Design review of the part shown in the three views and the two pictorial views. Dimensions are in mm from the part's minimum x, y and z. Give positions to 0.01 mm unless a question says otherwise; leave off trailing zeros. Write each loop counter-clockwise with the first axis right and the second up, starting at its lowest first coordinate (ties: lowest second). Pieces come first, ordered by that corner, then holes. Notation, with made-up numbers: M 42.5,31 L 85.5,31 A22 cw 85.5,44 Z; hole C -13,-19.5 d8. An arc over 180 degrees is marked long. Write item = value, one per line.
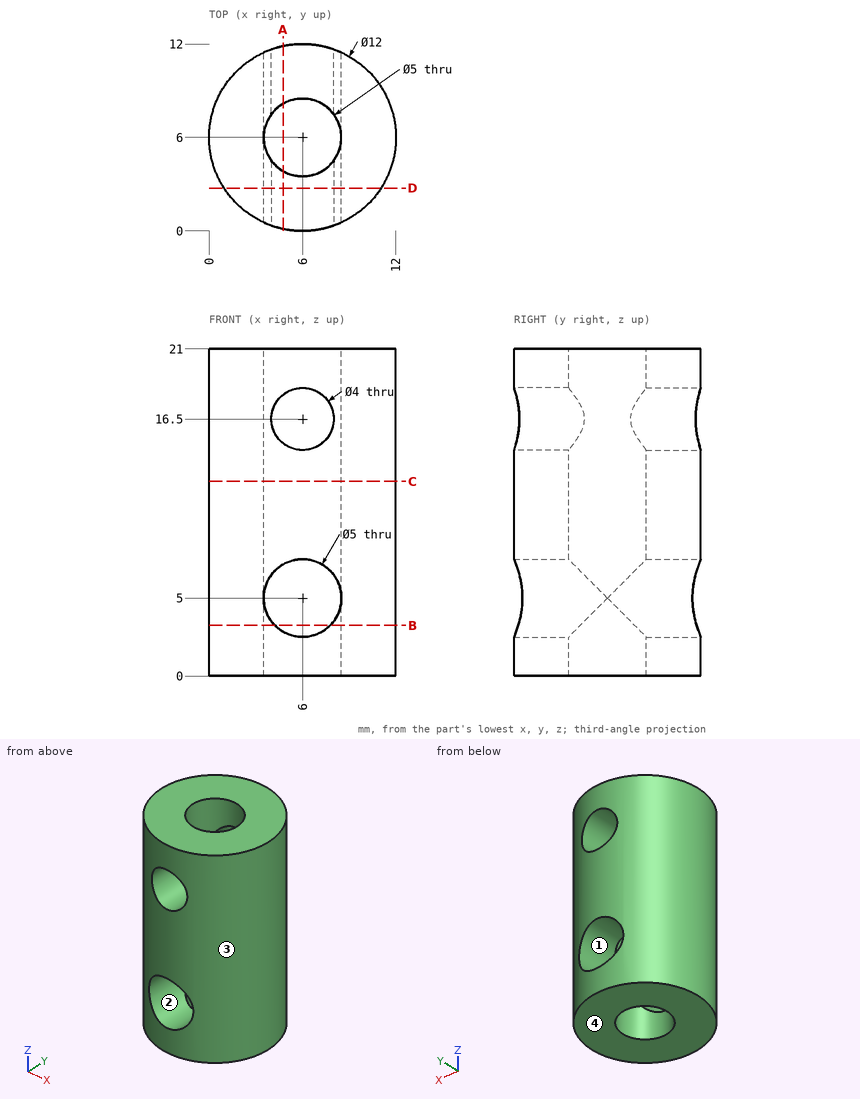
1. Insertion check: P1, Ø1.5, axis at x = 9.5, z = 7.5, coming from the -Y side; P2, Ø1, axis at y = 7, z = 6.5, coming from the -X side; P3, Ø2, axis at y = 8.5, z = 16.5, coming from the +X side. Each pin has a flat end and moves straight along its axis. Give the tip position at first contact, or say it passes through.
Responses:
P1 = 0.67
P2 = 0.02
P3 = 11.81
2. We need section C-C, the plane z = 12.5. Write out the cut boundary in (x, y), then the cut area to 3 significant figures.
Responses:
outline = C 6,6 d12; hole C 6,6 d5
area = 93.5 mm2
3. We need section B-B, the plane z = 3.25. Write out the cut boundary in (x, y).
Responses:
outline = M 4.21,0.27 L 4.21,4.25 A2.5 cw 4.21,7.75 L 4.21,11.73 A6 ccw Z; M 7.79,0.27 A6 ccw 7.79,11.73 L 7.79,7.75 A2.5 cw 7.79,4.25 Z
4. We need section D-D, the plane y = 2.75. Write out the cut boundary in (x, z).
Responses:
outline = M 0.96,0 L 11.04,0 L 11.04,21 L 0.96,21 Z; hole C 6,5 d5; hole C 6,16.5 d4
5. For line 1 along Z through (x, y) = (5, 1); line 2 along X through (y, z) = (6.75, 19); line 3 along Y through (x, z) = (6, 8.75), list the stretches that pass through material, from the lowest coordinate up. Write a range as from..to.
Responses:
line_1 = 0..2.71, 7.29..14.77, 18.23..21
line_2 = 0.05..3.62, 8.38..11.95
line_3 = 0..3.5, 8.5..12
6. We need section A-A, the plane x = 4.75. Write out the cut boundary in (y, z), then the cut area to 3 significant figures.
Responses:
outline = M 0.13,0 L 3.83,0 L 3.83,2.83 L 0.13,2.83 Z; M 0.13,7.17 L 3.83,7.17 L 3.83,14.94 L 0.13,14.94 Z; M 0.13,18.06 L 3.83,18.06 L 3.83,21 L 0.13,21 Z; M 8.17,0 L 11.87,0 L 11.87,2.83 L 8.17,2.83 Z; M 8.17,7.17 L 11.87,7.17 L 11.87,14.94 L 8.17,14.94 Z; M 8.17,18.06 L 11.87,18.06 L 11.87,21 L 8.17,21 Z
area = 100 mm2
7. The part is to be moulded in two halves that separate along X. For the marked faces 1, 2, 3 and 4, say which applies: +X half, -X half, draft (parallel to the pull), parting line (faces both ways), or undercut.
Responses:
face_1 = undercut
face_2 = undercut
face_3 = parting line
face_4 = draft
